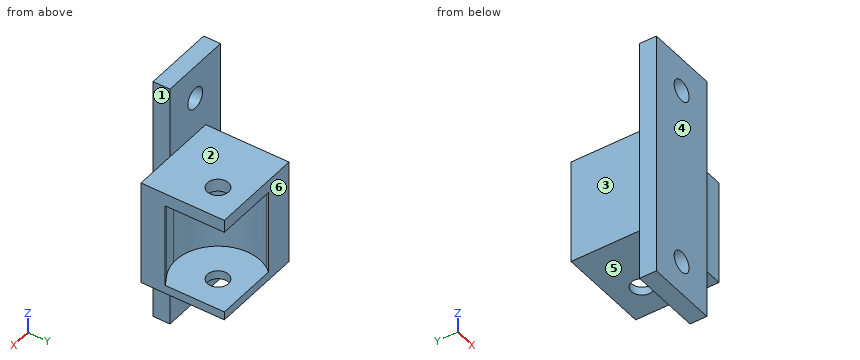
```python
from build123d import *

# Parameters (mm, degrees)
BOSS_EXTRUDE1_DEPTH = 27.94
SKETCH2_R           = 3.175
BOSS_EXTRUDE2_DEPTH = 2.54
BOSS_EXTRUDE3_START = 3.81
SKETCH3_W           = 27.611756562
SKETCH3_H           = 25.107614127
SKETCH3_R           = 3.175
BOSS_EXTRUDE3_DEPTH = 3.81
SKETCH4_W           = 21.59
SKETCH4_H           = 74.93
SKETCH4_R           = 3.175
BOSS_EXTRUDE4_DEPTH = 5.08


with BuildPart() as part:
    # Sketch1 → Boss-Extrude1 (new body)
    with BuildSketch(Plane.XY):
        with BuildLine():
            Line((-518.959059009, 348.633589309), (-527.727560082, 348.633589309))
            Line((-527.727560082, 348.633589309), (-527.727560082, 323.525975182))
            Line((-527.727560082, 323.525975182), (-500.11580352, 323.525975182))
            Line((-500.11580352, 323.525975182), (-500.11580352, 330.828951218))
            Line((-500.11580352, 330.828951218), (-503.31589155, 328.989459324))
            ThreePointArc((-503.31589155, 328.989459324), (-505.910190066, 327.86159111), (-508.689794246, 327.335975182))
            ThreePointArc((-508.689794246, 327.335975182), (-520.655570716, 333.67086151), (-520.107560082, 347.198990562))
            ThreePointArc((-520.107560082, 347.198990562), (-519.559291988, 347.937090778), (-518.959059009, 348.633589309))
        make_face()
    extrude(amount=-BOSS_EXTRUDE1_DEPTH)

    # Sketch2 → Boss-Extrude2 (add)
    with BuildSketch(Plane(origin=(0, 0, -25.4), x_dir=(-1, 0, 0), z_dir=(0, 0, -1))):
        with BuildLine():
            Line((500.11580352, 330.828951218), (500.11580352, 348.633589309))
            Line((500.11580352, 348.633589309), (518.959059009, 348.633589309))
            ThreePointArc((518.959059009, 348.633589309), (519.579835197, 332.088638139), (503.31589155, 328.989459324))
            Line((503.31589155, 328.989459324), (500.11580352, 330.828951218))
        make_face()
        with Locations(Location((509.64503004, 340, 0), (0, 0, 180))):
            Circle(SKETCH2_R, mode=Mode.SUBTRACT)
    extrude(amount=BOSS_EXTRUDE2_DEPTH)

    # Sketch3 → Boss-Extrude3 (add)
    with BuildSketch(Plane.XY.offset(BOSS_EXTRUDE3_START)):
        with Locations((-513.921681801, 336.079782246)):
            Rectangle(SKETCH3_W, SKETCH3_H)
        with Locations((-509.64503004, 340)):
            Circle(SKETCH3_R, mode=Mode.SUBTRACT)
    extrude(amount=-BOSS_EXTRUDE3_DEPTH)

    # Sketch4 → Boss-Extrude4 (add)
    with BuildSketch(Plane(origin=(0, 323.525975182, 0), x_dir=(1, 0, 0), z_dir=(0, 1, 0))):
        with Locations((-523.282560082, 12.065)):
            Rectangle(SKETCH4_W, SKETCH4_H)
        with Locations(Location((-523.282560082, -15.24, 0), (0, 0, 270))):
            Circle(SKETCH4_R, mode=Mode.SUBTRACT)
        with Locations(Location((-523.282560082, 39.37, 0), (0, 0, 270))):
            Circle(SKETCH4_R, mode=Mode.SUBTRACT)
    extrude(amount=-BOSS_EXTRUDE4_DEPTH)


solid = part.part
```
Could you check a few things on this model? Use its own coordinates, in mm. Face numbers are marked on the shaded views. A direction names the side the tool comes from. Give positions to 0.01 mm unless a question says otherwise; leave off trailing zeros. Loops run counter-clockwise (first coordinate to the right, second up) from the corner with the lowest first, then second, coordinate; pieces in that order, holes last. Notation, with made-up numbers: (83, 82.25) - (104, 82.25) arc R31 cw to (104, 107.25) - close; hole circle Ø9 at (34.25, 55.5). An arc over 180 degrees is marked (long way). Answer in a Markdown table with one row per item. Add a question column.
Q1. Which directions (+Z, -Z, +X, -X, +Y, -Y) give clear straight access to the entire face, cutting with the end or side of a thin tool? Please do the marked faces 1, 2 and 3.
Q2. For pin 1 (5 mm diameter, centred on x = -529, y = 339.5, fed in from -Z); pin 2 (6 mm diameter, centred on x = -509, y = 335.5, fed in from +Z); pin 3 (12 mm diameter, centred on y = 336.5, z = -10.5, fed in from -X), each with a flat end and sliding along its axis, tell me the tip position at first contact or that it passes through.
Q3. If we section it at A-A (z = 1.5): List the corners of the cut face in (x, y) for me (3 decimals).
Q4. Please list where these lines run through material, in increasing order: L1, parallel to X at y = 340, z = 1.6; L2, parallel to X at y = 321.4, z = 15.24; L3, parallel to Z at x = -504.5, y = 342.5. Write a range as from..to.
Q5. If we section it at D-D (z = -39.37): List the corners of the cut face in (x, y) for me.
Q6. We'd pull the mould along Y, two halves only. Please class the marked faces 4, 5 and 6: +Y half, -Y half, draft (parallel to the pull), parting line (faces both ways), or undercut.
Q7. If we section it at B-B (y = 340): List the corners of the cut face in (x, z) for me.
Q8. If we section it at C-C (x = -511): List the corners of the cut face in (y, z) for me.
The answers:
| question | item | result |
|---|---|---|
| 1 | face 1 | +Z, -Z, +X, -Y |
| 1 | face 2 | +Z, +X, -X, +Y |
| 1 | face 3 | +Z, -Z, -X, +Y |
| 2 | pin 1 | stops at z = -27.94 |
| 2 | pin 2 | stops at z = 3.81 |
| 2 | pin 3 | stops at x = -527.73 |
| 3 | outline | (-534.078, 318.446) - (-512.488, 318.446) - (-512.488, 323.526) - (-500.116, 323.526) - (-500.116, 348.634) - (-527.728, 348.634) - (-527.728, 323.526) - (-534.078, 323.526) - close; hole circle Ø6.35 at (-509.645, 340) |
| 4 | L1 | x = -527.73..-512.82, -506.47..-500.12 |
| 4 | L2 | x = -534.08..-526.46, -520.11..-512.49 |
| 4 | L3 | z = -27.94..-25.4, 0..3.81 |
| 5 | outline | (-534.08, 318.45) - (-526.46, 318.45) - (-526.46, 323.53) - (-534.08, 323.53) - close; (-520.11, 318.45) - (-512.49, 318.45) - (-512.49, 323.53) - (-520.11, 323.53) - close |
| 6 | face 4 | -Y half |
| 6 | face 5 | draft |
| 6 | face 6 | +Y half |
| 7 | outline | (-527.73, -27.94) - (-512.82, -27.94) - (-512.82, -25.4) - (-522.35, -25.4) - (-522.35, 0) - (-512.82, 0) - (-512.82, 3.81) - (-527.73, 3.81) - close; (-506.47, -27.94) - (-500.12, -27.94) - (-500.12, -25.4) - (-506.47, -25.4) - close; (-506.47, 0) - (-500.12, 0) - (-500.12, 3.81) - (-506.47, 3.81) - close |
| 8 | outline | (323.53, -27.94) - (337.13, -27.94) - (337.13, -25.4) - (327.37, -25.4) - (327.37, 0) - (337.13, 0) - (337.13, 3.81) - (323.53, 3.81) - close; (342.87, -27.94) - (348.63, -27.94) - (348.63, -25.4) - (342.87, -25.4) - close; (342.87, 0) - (348.63, 0) - (348.63, 3.81) - (342.87, 3.81) - close |
